The model under review builds one solid part; all positions refer to its coordinate system, in mm. Coordinates: 2 decimals unless noted, no trailing zeros. Order: outer loops, then holes, each group sorted by start corner. A loop starts at its lowest first (then second) coordinate and runs counter-clockwise, first axis right, second up. Notation, with made-up numbers: M 61,48.25 L 76,48.25 A14 ccw 76,54.25 Z; hole C 69,23.25 d11. An arc over 180 degrees is marked long. One line per item, written item: value.
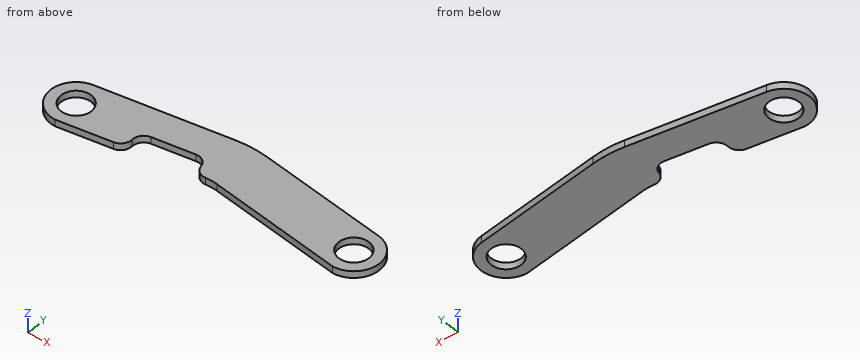
```python
from build123d import *

# Parameters (mm, degrees)
SKETCH1_R           = 14.2875
BOSS_EXTRUDE1_DEPTH = 6.35
FILLET2_R           = 101.6
FILLET4_R           = 10.16
FILLET5_R           = 10.16
FILLET6_R           = 10.16
FILLET7_R           = 43.18
FILLET8_R           = 10.16


with BuildPart() as part:
    # Sketch1 → Boss-Extrude1 (new body)
    with BuildSketch(Plane.XY):
        with BuildLine():
            Line((-265.377394078, 23.800923648), (-130.937, 43.529137522))
            Line((-130.937, 43.529137522), (3.490632878, 23.876188601))
            ThreePointArc((3.490632878, 23.876188601), (24.066463502, -1.749924149), (0, -24.13))
            Line((0, -24.13), (-130.937, -4.730862478))
            Line((-130.937, -4.730862478), (-144.883464555, -6.804936239))
            Line((-144.883464555, -6.804936239), (-147.640874452, 11.985780223))
            Line((-147.640874452, 11.985780223), (-205.570538861, 3.484995791))
            Line((-205.570538861, 3.484995791), (-202.760210881, -15.412181497))
            Line((-202.760210881, -15.412181497), (-261.874, -24.203395818))
            ThreePointArc((-261.874, -24.203395818), (-285.939994979, -1.829751605), (-265.377394078, 23.800923648))
        make_face()
        with Locations((-261.874, -0.073395818)):
            Circle(SKETCH1_R, mode=Mode.SUBTRACT)
        Circle(SKETCH1_R, mode=Mode.SUBTRACT)
    extrude(amount=BOSS_EXTRUDE1_DEPTH)

    # Fillet2
    fillet2_edges = [part.edges().sort_by_distance(p)[0] for p in [
        (-130.937, 43.529137522, 3.175),
    ]]
    fillet(fillet2_edges, radius=FILLET2_R)

    # Fillet4
    fillet4_edges = [part.edges().sort_by_distance(p)[0] for p in [
        (-147.640874452, 11.985780223, 3.175),
    ]]
    fillet(fillet4_edges, radius=FILLET4_R)

    # Fillet5
    fillet5_edges = [part.edges().sort_by_distance(p)[0] for p in [
        (-205.570538861, 3.484995791, 3.175),
    ]]
    fillet(fillet5_edges, radius=FILLET5_R)

    # Fillet6
    fillet6_edges = [part.edges().sort_by_distance(p)[0] for p in [
        (-202.760210881, -15.412181497, 3.175),
    ]]
    fillet(fillet6_edges, radius=FILLET6_R)

    # Fillet7
    fillet7_edges = [part.edges().sort_by_distance(p)[0] for p in [
        (-130.937, -4.730862478, 3.175),
    ]]
    fillet(fillet7_edges, radius=FILLET7_R)

    # Fillet8
    fillet8_edges = [part.edges().sort_by_distance(p)[0] for p in [
        (-144.883464555, -6.804936239, 3.175),
    ]]
    fillet(fillet8_edges, radius=FILLET8_R)


solid = part.part
```
(1) Insertion check: pin 1 Ø3 at (y, z) = (-2.5, 3) entering from -X; pin 2 Ø1 at (y, z) = (7, 5.5) entering from +X; pin 3 Ø2 at (x, z) = (-236.5, 1.5) entering from +Y. Each pin has a flat end and moves straight along its axis. Give the tip position at first contact, or say it passes through.
Geometry results:
pin 1: stops at x = -285.99
pin 2: stops at x = 23.24
pin 3: stops at y = 28.19
(2) For L1, parallel to X at y = 4, z = 5.75; L2, parallel to X at y = 12, z = 1.5; L3, parallel to X at y = 12.5, z = 4.5, list the stretches that pass through material, from the lowest coordinate up.
Geometry results:
L1: x = -285.66 to -275.57, -248.18 to -198.56, -146.7 to -13.72, 13.72 to 23.8
L2: x = -282.77 to -269.51, -254.23 to -7.75, 7.75 to 20.93
L3: x = -282.47 to -268.66, -255.09 to -6.92, 6.92 to 20.64
(3) We need section A-A, the plane z = 1.75. Count the separate pieces of the cut face and the enclosed holes in it, plus the area to 3 significant figures.
Geometry results:
separate pieces: 1
enclosed holes: 2
area: 12,100 mm2
(4) We need section C-C, the plane x = -52. State the section outline as (y, z) points.
Geometry results:
outline: M -16.43,0 L 31.99,0 L 31.99,6.35 L -16.43,6.35 Z
(5) We need section B-B, the plane x = -225. State the section outline as (y, z) points, plus the area to 3 significant figures.
Geometry results:
outline: M -18.72,0 L 29.73,0 L 29.73,6.35 L -18.72,6.35 Z
area: 308 mm2
